Geometry check sheet. Reference: the model listing, model coordinates, mm. Face numbers are marked on the shaded views. A direction names the side the tool comes from. Coordinates: 2 decimals unless noted, no trailing zeros. Write each loop counter-clockwise with the first axis right and the second up, starting at its lowest first coordinate (ties: lowest second). Pieces come first, ordered by that corner, then holes. Notation, with made-up numbers: (22, 53) -> (59, 53) arc R34 ccw to (59, 88) -> close; hole circle Ø9 at (82.25, 26). An arc over 180 degrees is marked (long way). Answer in a Markdown table with one row per item. Add a question column.
1. Cross-section at A-A on x = -19. Record the cut outline in (y, z), and give its area (3 significant figures).
2. Scan lines: L1, parallel to Y at x = -55, z = 0; L2, parallel to Z at x = -54.5, y = 24; L3, parallel to X at y = 10, z = -7.5. Record each from-to range of solid material in increasing order. Write a range as from..to.
3. Depth check by flat-ended pin: P1, Ø2.5, axis at x = 9, y = 21.5, coming from the -Z side; P2, Ø6, axis at x = -11.5, z = 16.5, coming from the -Y side; P3, Ø20, axis at y = 32.85, z = 0, coming from the +X side. Enter the tip coordinate at first touch or a pass-through.
4. Cross-section at B-B on y = -13.5. Record the cut outline in (x, z) (3 decimals), and give its area (3 significant figures).
5. Mould release check, pull along X, two halves, no side actions. Record for the marked faces 4, 5 and 6: pulls with the +X half, pulls with the -X half, needs draft (parallel to the pull), parting line crosses it, or undercut.
6. Set-up check for the marked faces 1, 2 and 3: record each of +Z, -Z, +X, -X, +Y, -Y from which the full face is reachable in a straight line by a thin tool's end or side.
7. Cross-section at D-D on y = 5. Record the cut outline in (x, z), and give its area (3 significant figures).
8. Cross-section at C-C on z = 18. Record the cut outline in (x, y).
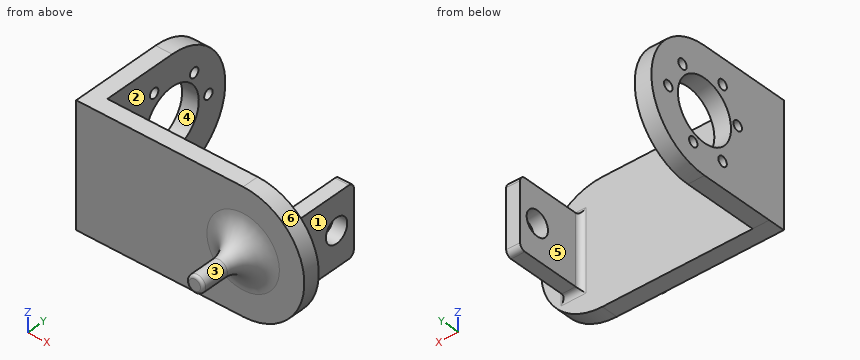
```python
from build123d import *

# Parameters (mm, degrees)
BOSS_EXTRUDE1_DEPTH = 6
BOSS_EXTRUDE2_DEPTH = 6
SKETCH3_R           = 11
SKETCH3_R_2         = 1.75
CUT_EXTRUDE1_DEPTH  = 6
SKETCH4_R           = 3.025
BOSS_EXTRUDE3_DEPTH = 20
FILLET1_R           = 10
FILLET2_R           = 1
SKETCH5_W           = 5
SKETCH5_H           = 25
BOSS_EXTRUDE4_DEPTH = 25
CUT_EXTRUDE2_REACH  = 95.817
SKETCH6_R           = 4.419567015
FILLET3_R           = 2


with BuildPart() as part:
    # Sketch1 → Boss-Extrude1 (new body)
    with BuildSketch(Plane(origin=(0, 0, 0), x_dir=(1, 0, 0), z_dir=(0, 1, 0))):
        with BuildLine():
            Line((0, -22), (-60, -22))
            Line((-60, -22), (-60, 22))
            Line((-60, 22), (0, 22))
            ThreePointArc((0, 22), (22, 0), (0, -22))
        make_face()
    extrude(amount=BOSS_EXTRUDE1_DEPTH)

    # Sketch2 → Boss-Extrude2 (add)
    with BuildSketch(Plane.ZY.offset(60)):
        with BuildLine():
            Line((-22, 6), (-21.999999972, 32.847291098))
            ThreePointArc((-21.999999972, 32.847291098), (-0.000557287, 54.848405664), (22, 32.848405671))
            Line((22, 32.848405671), (22, 6))
            Line((22, 6), (-22, 6))
        make_face()
    extrude(amount=-BOSS_EXTRUDE2_DEPTH)

    # Sketch3 → Cut-Extrude1 (cut)
    with BuildSketch(Plane.ZY.offset(60)):
        with Locations((0, 32.848405671)):
            Circle(SKETCH3_R)
        with Locations((0, 47.848405671)):
            Circle(SKETCH3_R_2)
        with Locations((12.990381057, 25.348405671)):
            Circle(SKETCH3_R_2)
        with Locations((-12.990381057, 25.348405671)):
            Circle(SKETCH3_R_2)
        with Locations((10.623744158, 41.966303458)):
            Circle(SKETCH3_R_2)
        with Locations((2.584459033, 19.089024453)):
            Circle(SKETCH3_R_2)
        with Locations((-13.208203192, 37.489889102)):
            Circle(SKETCH3_R_2)
    extrude(amount=-CUT_EXTRUDE1_DEPTH, mode=Mode.SUBTRACT)

    # Sketch4 → Boss-Extrude3 (add)
    with BuildSketch(Plane.XZ):
        with Locations(Location((0, 0, 0), (0, 0, 90))):
            Circle(SKETCH4_R)
    extrude(amount=BOSS_EXTRUDE3_DEPTH)

    # Fillet1
    fillet1_edges = [part.edges().sort_by_distance(p)[0] for p in [
        (0, 0, -3.025),
    ]]
    fillet(fillet1_edges, radius=FILLET1_R)

    # Fillet2
    fillet2_edges = [part.edges().sort_by_distance(p)[0] for p in [
        (0, -20, -3.025),
    ]]
    fillet(fillet2_edges, radius=FILLET2_R)

    # Sketch5 → Boss-Extrude4 (add)
    with BuildSketch(Plane(origin=(0, 6, 0), x_dir=(1, 0, 0), z_dir=(0, 1, 0))):
        with Locations((10.364576522, 0)):
            Rectangle(SKETCH5_W, SKETCH5_H)
    extrude(amount=BOSS_EXTRUDE4_DEPTH)

    # Sketch6 → Cut-Extrude2 (cut, up to next)
    with BuildSketch(Plane(origin=(12.864576522, 0, 0), x_dir=(0, 0, -1), z_dir=(1, 0, 0)), mode=Mode.PRIVATE) as cut_extrude2_sk1:
        with Locations((0, 23.878810585)):
            Circle(SKETCH6_R)
    cut_extrude2_tool1 = extrude(cut_extrude2_sk1.sketch, amount=-CUT_EXTRUDE2_REACH, mode=Mode.PRIVATE) & part.part
    add(cut_extrude2_tool1.solids().sort_by_distance((12.864577, 23.878811, 0))[0], mode=Mode.SUBTRACT)

    # Fillet3
    fillet3_edges = [part.edges().sort_by_distance(p)[0] for p in [
        (12.864576522, 6, 0),
        (10.364576522, 6, -12.5),
        (7.864576522, 6, 0),
        (10.364576522, 6, 12.5),
        (10.364576522, 31, -12.5),
        (10.364576522, 31, 12.5),
    ]]
    fillet(fillet3_edges, radius=FILLET3_R)


solid = part.part
```
Results found:
| question | item | result |
|---|---|---|
| 1 | outline | (0, -22) -> (6, -22) -> (6, 22) -> (0, 22) -> close |
| 1 | area | 264 mm^2 |
| 2 | L1 | y = 0..21.85, 43.85..46.1, 49.6..54.85 |
| 2 | L2 | z = -22..-14.11, -11.87..-6.53, 6.53..11.87, 14.11..22 |
| 2 | L3 | x = -60..-54, 7.86..12.86 |
| 3 | P1 | stops at z = -12.5 |
| 3 | P2 | stops at y = 0 |
| 3 | P3 | stops at x = 12.86 |
| 4 | outline | circle Ø6.05 at (0, 0) |
| 4 | area | 28.7 mm^2 |
| 5 | face 4 | needs draft |
| 5 | face 5 | undercut |
| 5 | face 6 | pulls with the +X half |
| 6 | face 1 | +Z, -Z, +X, +Y |
| 6 | face 2 | +Z, -Z, +Y |
| 6 | face 3 | -Y |
| 7 | outline | (-60, -22) -> (0, -22) arc R22 ccw to (0, 22) -> (-60, 22) -> close |
| 7 | area | 3,400 mm^2 |
| 8 | outline | (-60, 0) -> (12.65, 0) -> (12.65, 6) -> (-54, 6) -> (-54, 45.5) -> (-60, 45.5) -> close |
